Can you work these out from the model? Positions are in its coordinate system, mm. Face numbers are marked on the shaded views. A direction names the side the tool comes from. Coordinates: 2 decimals unless noted, no trailing zeros. Loops run counter-clockwise (first coordinate to the right, second up) from the corner with the lowest first, then second, coordinate; pieces in that order, holes last.
```python
from build123d import *

# Parameters (mm, degrees)
BOSS_EXTRUDE1_DEPTH = 20
SKETCH4_W           = 10
SKETCH4_H           = 4
BOSS_EXTRUDE2_DEPTH = 6
SKETCH5_R           = 1
CUT_EXTRUDE1_DEPTH  = 3
CIRPATTERN1_COUNT   = 4


with BuildPart() as part:
    # Sketch1 → Boss-Extrude1 (new body)
    with BuildSketch(Plane.XY):
        with BuildLine():
            Line((-8.5, -10.5), (8.5, -10.5))
            ThreePointArc((8.5, -10.5), (9.914213562, -9.914213562), (10.5, -8.5))
            Line((10.5, -8.5), (10.5, 8.5))
            ThreePointArc((10.5, 8.5), (9.914213562, 9.914213562), (8.5, 10.5))
            Line((8.5, 10.5), (-8.5, 10.5))
            ThreePointArc((-8.5, 10.5), (-9.914213562, 9.914213562), (-10.5, 8.5))
            Line((-10.5, 8.5), (-10.5, -8.5))
            ThreePointArc((-10.5, -8.5), (-9.914213562, -9.914213562), (-8.5, -10.5))
        make_face()
    extrude(amount=BOSS_EXTRUDE1_DEPTH)

    # Sketch3 → Revolve1 (revolve)
    with BuildSketch(Plane(origin=(0, 0, 0), x_dir=(0, 0, -1), z_dir=(1, 0, 0))):
        Polygon((-20, 10.5), (-20, 0), (-25, 0), (-25, 5.035898385), (-31, 8.5), (-31, 10.5), align=None)
    revolve(axis=Axis((0, 0, 20), (0, 0, 1)))

    # Sketch4 → Boss-Extrude2 (add)
    with BuildSketch(Plane(origin=(0, 0, 0), x_dir=(-1, 0, 0), z_dir=(0, 0, -1))):
        with Locations((0, -7.5)):
            Rectangle(SKETCH4_W, SKETCH4_H)
    extrude(amount=BOSS_EXTRUDE2_DEPTH)

    # Sketch5 → Cut-Extrude1 (cut)
    with BuildSketch(Plane.ZY.offset(10.5)):
        with Locations((18, 6)):
            Circle(SKETCH5_R)
        with Locations((18, -6)):
            Circle(SKETCH5_R)
    cut_extrude1 = extrude(amount=-CUT_EXTRUDE1_DEPTH, mode=Mode.SUBTRACT)

    # CirPattern1: Cut-Extrude1 ×4 about axis
    cirpattern1_axis = Axis((0, 0, 0), (0, 0, 1))
    for i in range(1, CIRPATTERN1_COUNT):
        add(cut_extrude1.rotate(cirpattern1_axis, i * 360 / CIRPATTERN1_COUNT), mode=Mode.SUBTRACT)


solid = part.part
```
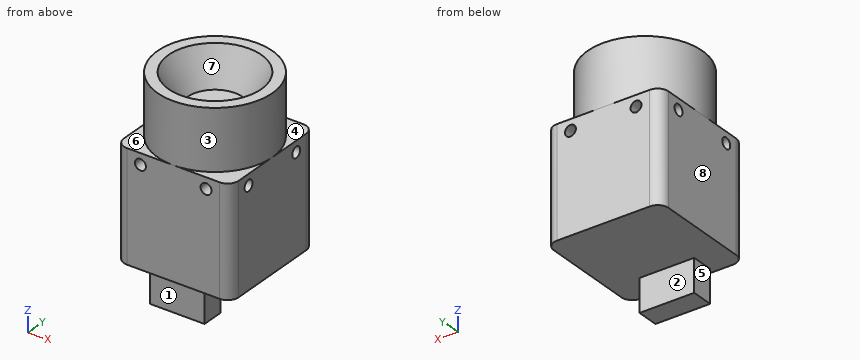
Item 1: Suppose I cut it at A-A, the plane y = 9. Please give me the cut outline in (x, z).
Results are:
outline: (-10.44, 0) - (10.44, 0) - (10.44, 20) - (5.41, 20) - (5.41, 31) - (-5.41, 31) - (-5.41, 20) - (-10.44, 20) - close; hole circle Ø2 at (-6, 18); hole circle Ø2 at (6, 18)
Item 2: On a 3-axis mill with a long thin cutter (end or side, diameter ignored), from which of +Z, -Z, +X, -X, +Y, -Y can I reach the whole of each face in a straight line? I mean the marked faces 1, 2, 3, 4 and 5. Say none if no direction works.
Results are:
face 1: -Z, +X, -X, -Y
face 2: -Z, +X, -X, +Y
face 3: +Z
face 4: +Z, +X, +Y
face 5: -Z, -X, +Y, -Y
Item 3: I need wall thicknesses on line 1 along Y through (x, z) = (-8.9, 18); line 2 along Z through (x, y) = (1.75, -1.25); line 3 along X through (y, z) = (9.7, 18). Which ranges of each line are inside material? Lowest first, please.
Results are:
line 1: y = -10.46 to -7, -5 to 5, 7 to 10.46
line 2: z = 0 to 25
line 3: x = -10.1 to -7, -5 to 5, 7 to 10.1
Item 4: Suppose I cut it at B-B, the plane z = 20.5. Please give me the cut outline in (x, y), plus the area to 3 significant figures.
Results are:
outline: circle Ø21 at (0, 0)
area: 346 mm2
Item 5: We'd pull the mould along X, two halves only. Please class the marked faces 6, 7 and 8: +X half, -X half, draft (parallel to the pull), parting line (faces both ways), or undercut.
Results are:
face 6: draft
face 7: undercut
face 8: -X half
Item 6: I'm going to push flat-ended pins straight in: P1, Ø1.8, axis at y = -6, z = 18, coming from the +X side; P2, Ø1.6, axis at y = -6, z = 18, coming from the -X side; P3, Ø10.5, axis at x = 3, y = 0.5, coming from the -Z side. Where does each tip first touch, or does it pass through?
Results are:
P1: stops at x = 7.5
P2: stops at x = -7.5
P3: stops at z = 0
